from build123d import *

# Parameters (mm, degrees)
F0_W     = 130.505652
F0_H     = 74.890166
F0_R     = 5.943332
F0_R_2   = 5.936545
F1_DEPTH = 50.8
F3_DEPTH = 56.642
F4_DEPTH = 111.252


with BuildPart() as f1:
    # F0 (on Top) → F1 (new body)
    with BuildSketch(Plane.XY):
        Rectangle(F0_W, F0_H)
        with Locations((-56.619376, 0)):
            Circle(F0_R, mode=Mode.SUBTRACT)
        with Locations((57.221707, 0)):
            Circle(F0_R_2, mode=Mode.SUBTRACT)
    extrude(amount=F1_DEPTH)

    # F2 (on Front) → F3 (join, symmetric)
    with BuildSketch(Plane.XZ):
        with BuildLine():
            Line((-26.310177, 51.006424), (-38.046643, 51.006424))
            ThreePointArc((-38.046643, 51.006424), (0.00796, 13.051229), (38.046678, 51.022345))
            Line((38.046678, 51.022345), (26.310227, 51.022345))
            ThreePointArc((26.310227, 51.022345), (0.00796, 24.787647), (-26.310177, 51.006424))
        make_face()
    extrude(amount=F3_DEPTH, both=True)

    # F3_face (on face) → F4 (cut, symmetric)
    with BuildSketch(Plane(origin=(0, 37.445083, 39.770332), x_dir=(-1, 0, 0), z_dir=(0, 1, 0))):
        with BuildLine():
            ThreePointArc((-26.308649, 11.029668), (0, -14.982687), (26.308649, 11.029668))
            Line((26.308649, 11.029668), (-26.308649, 11.029668))
        make_face()
    extrude(amount=F4_DEPTH, both=True, mode=Mode.SUBTRACT)


solid = f1.part
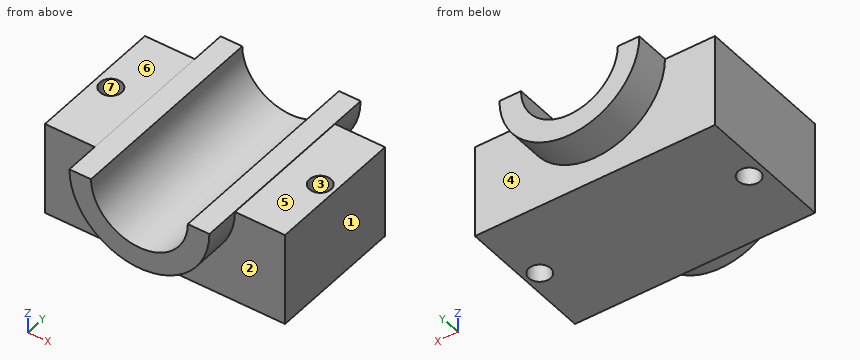
Source: CAD feature listing. Evaluate the final solid. Frame: model axes, mm. Face numbers are marked on the shaded views. A direction names the side the tool comes from. Coordinates: 2 decimals unless noted, no trailing zeros. Loops run counter-clockwise (first coordinate to the right, second up) from the corner with the lowest first, then second, coordinate; pieces in that order, holes last. Notation, with made-up numbers: (-10, -37) - (9, -37) arc R31 ccw to (9, -4) - close; hole circle Ø3 at (49, -10). An arc over 180 degrees is marked (long way). One line per question, with ' | ' between items.
1) Section D-D, the plane z = 8.5. Return loops of the section in (x, y).
Report:
outline: (-65.25, -37.45) - (65.25, -37.45) - (65.25, 37.45) - (-65.25, 37.45) - close; hole circle Ø11.89 at (-56.62, 0); hole circle Ø11.87 at (57.22, 0)
2) First-contact query: P1, Ø13.5, axis at x = -57.5, y = -3, coming from the +Z side; P2, Ø3, axis at x = 20.5, y = 44.5, coming from the -Z side; P3, Ø12, axis at x = -51.5, z = 22.5, coming from the +Y side. Flat tips, straight axial feed; report the tip coordinate or a pass-through.
Report:
P1: stops at z = 50.8 | P2: stops at z = 18.14 | P3: stops at y = 37.45
3) Line query: line 1 along X through (y, z) = (-2.5, 8.5); line 2 along Y through (x, z) = (-57, 42.5); line 3 along Z through (x, y) = (47, -10). Output: solid intervals per line, ascending.
Report:
line 1: x = -65.25 to -62.01, -51.23 to 51.84, 62.61 to 65.25 | line 2: y = -37.45 to -5.93, 5.93 to 37.45 | line 3: z = 0 to 50.8
4) Section C-C, the plane x = 0. Return loops of the section in (y, z).
Report:
outline: (-56.64, 13.05) - (-37.45, 13.05) - (-37.45, 0) - (37.45, 0) - (37.45, 13.05) - (56.64, 13.05) - (56.64, 24.79) - (-56.64, 24.79) - close
5) Pull-direction query (X, two-part tool) for the marked faces 1, 2 and 3; classes: released by +X, released by -X, zero draft, split by the parting line, or undercut.
Report:
face 1: released by +X | face 2: zero draft | face 3: undercut
6) Section B-B, the plane z = 37. Return loops of the section in (x, y).
Report:
outline: (-65.25, -37.45) - (-35.34, -37.45) - (-35.34, -56.64) - (-22.21, -56.64) - (-22.21, 56.64) - (-35.34, 56.64) - (-35.34, 37.45) - (-65.25, 37.45) - close; (22.21, -56.64) - (35.34, -56.64) - (35.34, -37.45) - (65.25, -37.45) - (65.25, 37.45) - (35.34, 37.45) - (35.34, 56.64) - (22.21, 56.64) - close; hole circle Ø11.89 at (-56.62, 0); hole circle Ø11.87 at (57.22, 0)
7) Set-up query: the marked faces 4, 5, 6 and 7. Return all of +Z, -Z, +X, -X, +Y, -Y with unobstructed straight access to the full face (end or side cutting, diameter ignored); none if empty.
Report:
face 4: -Z, +Y | face 5: +Z, +X, +Y, -Y | face 6: +Z, -X, +Y, -Y | face 7: +Z, -Z
8) Section A-A, the plane y = 0. Return loops of the section in (x, z), then the cut area to 3 significant figures.
Report:
outline: (-65.25, 0) - (-62.56, 0) - (-62.56, 50.8) - (-65.25, 50.8) - close; (-50.68, 0) - (51.29, 0) - (51.29, 50.8) - (38.05, 50.8) arc R38.05 ccw to (38.05, 51.02) - (26.31, 51.02) arc R26.31 cw to (-26.31, 51.01) - (-38.05, 51.01) arc R38.05 ccw to (-38.05, 50.8) - (-50.68, 50.8) - close; (63.16, 0) - (65.25, 0) - (65.25, 50.8) - (63.16, 50.8) - close | area: 4,360 mm²
